```python
from build123d import *

# Parameters (mm, degrees)
SKETCH1_W           = 28
SKETCH1_H           = 39
BOSS_EXTRUDE1_DEPTH = 2.5
SKETCH2_W           = 28
SKETCH2_H           = 2.5
BOSS_EXTRUDE2_DEPTH = 46.5
SKETCH3_W           = 5.5
SKETCH3_H           = 5.5
SKETCH3_R           = 1.4
BOSS_EXTRUDE3_DEPTH = 28


with BuildPart() as part:
    # Sketch1 → Boss-Extrude1 (new body)
    with BuildSketch(Plane(origin=(0, 0, 0), x_dir=(1, 0, 0), z_dir=(0, 1, 0))):
        Rectangle(SKETCH1_W, SKETCH1_H)
    extrude(amount=BOSS_EXTRUDE1_DEPTH)

    # Sketch2 → Boss-Extrude2 (add)
    with BuildSketch(Plane(origin=(0, 2.5, 0), x_dir=(1, 0, 0), z_dir=(0, 1, 0))):
        with Locations((0, 18.25)):
            Rectangle(SKETCH2_W, SKETCH2_H)
    extrude(amount=BOSS_EXTRUDE2_DEPTH)

    # Sketch3 → Boss-Extrude3 (add)
    with BuildSketch(Plane(origin=(14, 0, 0), x_dir=(0, 0, -1), z_dir=(1, 0, 0))):
        with Locations((22.25, 12.75)):
            Rectangle(SKETCH3_W, SKETCH3_H)
        with Locations((22.5, 12.75)):
            Circle(SKETCH3_R, mode=Mode.SUBTRACT)
    extrude(amount=-BOSS_EXTRUDE3_DEPTH)


solid = part.part
```
Geometry check sheet. Reference: the model listing, model coordinates, mm. A direction names the side the tool comes from. Round coordinates to 2 decimals unless told otherwise and drop trailing zeros. Loops run counter-clockwise (first coordinate to the right, second up) from the corner with the lowest first, then second, coordinate; pieces in that order, holes last. Notation, with made-up numbers: (61, -4.5) - (106, -4.5) arc R17 cw to (106, 22.5) - close; hole circle Ø7 at (-32.75, -11.75). An arc over 180 degrees is marked (long way). Use a Markdown table: item, result.
Q1. Cross-section at A-A on z = -22.5. Record the cut outline in (x, y), plus the area to 3 significant figures.
Solutions:
| item | result |
|---|---|
| outline | (-14, 10) - (14, 10) - (14, 11.35) - (-14, 11.35) - close; (-14, 14.15) - (14, 14.15) - (14, 15.5) - (-14, 15.5) - close |
| area | 75.6 mm2 |
Q2. Go/stop test with flat-tipped pins: P1, Ø1, axis at x = -10.5, z = -11, coming from the +Y side; P2, Ø12, axis at x = -5, y = 11.5, coming from the +Z side; P3, Ø6, axis at x = -4.5, z = -23.5, coming from the -Y side. Record where each tip stops, or that it passes through.
Solutions:
| item | result |
|---|---|
| P1 | stops at y = 2.5 |
| P2 | stops at z = -17 |
| P3 | stops at y = 10 |
Q3. Material ranges on line 1 (Y direction, x = -5.5, z = -22.5); line 2 (Y direction, x = -4.5, z = 5.5); line 3 (Z direction, x = -2.5, y = 20.5), recorded low to high.
Solutions:
| item | result |
|---|---|
| line 1 | y = 10 to 11.35, 14.15 to 15.5 |
| line 2 | y = 0 to 2.5 |
| line 3 | z = -19.5 to -17 |
Q4. Access from +Z, -Z, +X, -X, +Y, -Y to the whole of each face (thin tool, end or side, straight path). Record for faces 4 (the flat face through (-14, 17.1, -17.5)), 5 (the flat face through (0, 49, -18)), 6 (the flat face through (0, 15.5, -22)), 7 (the flat face through (0, 10, -22)), 8 (the flat face through (0, 2.5, 1)).
Solutions:
| item | result |
|---|---|
| face 4 | +Z, -Z, -X, +Y, -Y |
| face 5 | +Z, -Z, +X, -X, +Y |
| face 6 | -Z, +X, -X, +Y |
| face 7 | -Z, +X, -X, -Y |
| face 8 | +Z, +X, -X, +Y |
Q5. Cross-section at B-B on y = 12.75. Record the cut outline in (x, z), plus the area to 3 significant figures.
Solutions:
| item | result |
|---|---|
| outline | (-14, -25) - (14, -25) - (14, -23.9) - (-14, -23.9) - close; (-14, -21.1) - (14, -21.1) - (14, -17) - (-14, -17) - close |
| area | 146 mm2 |
Q6. Cross-section at D-D on z = -9.5. Record the cut outline in (x, y).
Solutions:
| item | result |
|---|---|
| outline | (-14, 0) - (14, 0) - (14, 2.5) - (-14, 2.5) - close |
Q7. Cross-section at C-C on x = 5. Record the cut outline in (y, z).
Solutions:
| item | result |
|---|---|
| outline | (0, -19.5) - (10, -19.5) - (10, -25) - (15.5, -25) - (15.5, -19.5) - (49, -19.5) - (49, -17) - (2.5, -17) - (2.5, 19.5) - (0, 19.5) - close; hole circle Ø2.8 at (12.75, -22.5) |
Q8. Draft check along Z on faces 1 (the cylindrical face through (0.2, 13.9, -23.3)), 2 (the flat face through (0, 0, 0)), 3 (the flat face through (0, 1, 19.5)). Enter one of: released by +Z, released by -Z, zero draft, split by the parting line, or undercut.
Solutions:
| item | result |
|---|---|
| face 1 | undercut |
| face 2 | zero draft |
| face 3 | released by +Z |
